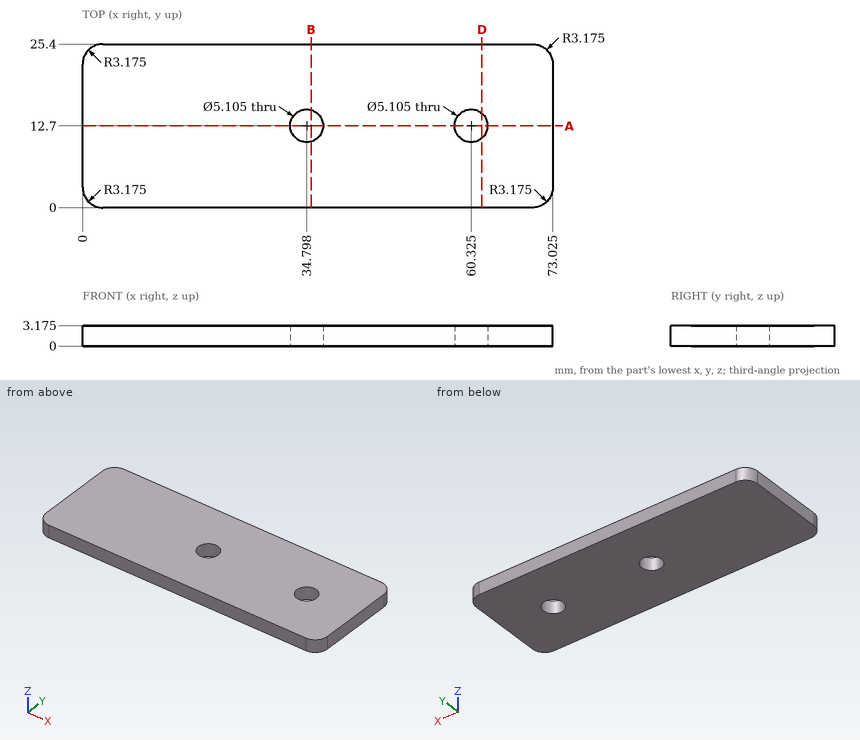
Check sheet for the drawn part. Datum: minimum x, y, z corner. Units: mm. Round coordinates to 2 decimals unless told otherwise and drop trailing zeros. Order: outer loops, then holes, each group sorted by start corner. A loop starts at its lowest first (then second) coordinate and runs counter-clockwise, first axis right, second up. Notation, with made-up numbers: M 31,22.5 L 54,22.5 A18 cw 54,57.5 Z; hole C -21,7 d8. An arc over 180 degrees is marked long. Write each question's results on one line, items separated by ' | '. Start each with the question number.
1. Go/stop test with a flat-tipped pin: P1, Ø6.5, axis at x = 60.325, y = 12.7, coming from the +Z side (3 decimals). Record where the tip stops, or that it passes through.
2. Material ranges on L1, parallel to X at y = 12, z = 0.25 (1 decimal); L2, parallel to Y at x = 33, z = 0.8; L3, parallel to X at y = 1.75, z = 0.4, recorded low to high. Write a range as from..to.
3. Cross-section at A-A on y = 12.7. Give the number of separate pieces and of enclosed holes in the cut face.
4. Cross-section at D-D on x = 62. Record the boundary of the cut face in (y, z) (1 decimal).
5. Cross-section at B-B on x = 35.5. Record the boundary of the cut face in (y, z) (1 decimal).
Resolved:
1) P1: z = 3.175
2) L1: 0..32.3, 37.3..57.9, 62.8..73 | L2: 0..10.89, 14.51..25.4 | L3: 0.34..72.69
3) separate pieces: 3 | enclosed holes: 0
4) outline: M 0,0 L 10.8,0 L 10.8,3.2 L 0,3.2 Z; M 14.6,0 L 25.4,0 L 25.4,3.2 L 14.6,3.2 Z
5) outline: M 0,0 L 10.2,0 L 10.2,3.2 L 0,3.2 Z; M 15.2,0 L 25.4,0 L 25.4,3.2 L 15.2,3.2 Z
